Autodesk Inventor part; units mm, degrees
ref_plane "YZ Plane" through (0, 0, 0) normal (1, 0, 0) x (0, 1, 0)
ref_plane "XZ Plane" through (0, 0, 0) normal (0, 1, 0) x (-1, 0, 0)
ref_plane "XY Plane" through (0, 0, 0) normal (0, 0, 1) x (1, 0, 0)
sketch "Sketch1" plane through (0, 0, 0) normal (0, 1, 0) x (-1, 0, 0)
  line L0 (5, 11.4699) -> (-5, 11.4699)
  line L1 (-5, 11.4699) -> (-5, -11.5301)
  line L2 (-5, -11.5301) -> (5, -11.5301)
  line L3 (5, -11.5301) -> (5, 11.4699)
  line L4 (0, 11.4699) -> (0, -11.5301) construction
  line L5 (5, 0.0301) -> (-5, -0.0301) construction
  point P0 (0, 0)
  point P1 (0, 0)
  point P2 (0, -0.0301)
  dimension "d0" = 10
  dimension "d1" = 23
extrude "Extrusion1" add sketch "Sketch1" along normal blind 13
sketch "Sketch4" plane through (-5, 0, 11.4699) normal (0, 0, 1) x (1, 0, 0)
  circle A0 centre (5, 0) radius 4
  dimension "d11" = 8
hole "Hole1" at (0, 0, 11.4699) direction (0, 0, -1) diameter 8 end through all
properties part number "arm_block"
Design review of the part built by this model. Coordinates are the model's own, in mm. Give positions to 0.01 mm unless a question says otherwise; leave off trailing zeros. Order: outer loops, then holes, each group sorted by start corner. A loop starts at its lowest first (then second) coordinate and runs counter-clockwise, first axis right, second up. Notation, with made-up numbers: (-39.5, 89.25) - (-0.5, 89.25) arc R23 cw to (-0.5, 110.25) - close; hole circle Ø11 at (15.25, 18.25). An arc over 180 degrees is marked (long way). Use a Markdown table: item, result. Add a question column.
(1) Add section A-A on y = 3.75. Give the boundary of the cut face in (x, z).
(2) Add section D-D on x = 2.75. Give the boundary of the cut face in (y, z), then the cut area to 3 significant figures.
(3) Clearance check with a flat-ended pin moving along its axis: P1, Ø1.5, axis at x = 3.5, z = 1.5, coming from the -Y side. State where the tip first meets the part, or that it passes through.
(4) Add section C-C on x = -1.75. Give the boundary of the cut face in (y, z).
(5) Wall thickness on probe 1 along X at (y, z) = (3.25, 6.5); probe 2 along Y at (x, z) = (0.25, 7.5); probe 3 along Y at (x, z) = (-2.25, -5.75): over which ranges is each line inside the solid? List them lowest first. Write a range as [from, to].
(6) Add section B-B on z = -4.75. Give the boundary of the cut face in (x, y), then the cut area to 3 significant figures.
Report:
| question | item | result |
|---|---|---|
| 1 | outline | (-5, -11.53) - (-1.39, -11.53) - (-1.39, 11.47) - (-5, 11.47) - close; (1.39, -11.53) - (5, -11.53) - (5, 11.47) - (1.39, 11.47) - close |
| 2 | outline | (2.9, -11.53) - (13, -11.53) - (13, 11.47) - (2.9, 11.47) - close |
| 2 | area | 232 mm² |
| 3 | P1 | stops at y = 0 |
| 4 | outline | (3.6, -11.53) - (13, -11.53) - (13, 11.47) - (3.6, 11.47) - close |
| 5 | probe 1 | x = [-5, -2.33], [2.33, 5] |
| 5 | probe 2 | y = [3.99, 13] |
| 5 | probe 3 | y = [3.31, 13] |
| 6 | outline | (-5, 0) - (-4, 0) arc R4 cw to (4, 0) - (5, 0) - (5, 13) - (-5, 13) - close |
| 6 | area | 105 mm² |
